The listing builds one solid part. Answer for the finished solid, in the listing's coordinates (mm). A direction names the side the tool comes from. Give positions to 0.01 mm unless a question says otherwise; leave off trailing zeros. Write each loop counter-clockwise with the first axis right and the second up, starting at its lowest first coordinate (ties: lowest second). Pieces come first, ordered by that corner, then holes. Notation, with made-up numbers: (-7, -14) - (16, -14) arc R31 cw to (16, 12) - close; hole circle Ø1 at (0, 5). An arc over 180 degrees is marked (long way). One line per item, written item: value. Start each with the question number.
from build123d import *

# Parameters (mm, degrees)
F1_DEPTH      = 57.15
F1_DEPTH_BACK = 57.15
F2_R          = 6.35
F3_R          = 6.35
F4_R          = 9.525
F5_R          = 4.445
F6_DEPTH      = 101.346
F6_DEPTH_BACK = 150.622
F7_R          = 4.7625
F8_DEPTH      = 25.4
F8_DEPTH_BACK = 25.4
F9_R          = 25.4


with BuildPart() as f1:
    # F0 (on Front) → F1 (new body, two sides)
    with BuildSketch(Plane.XZ) as f1_sk:
        Polygon((-22.225, 0), (0, 0), (22.225, 0), (22.225, 76.2), (19.05, 76.2), (19.05, 3.175), (0, 3.175), (-19.05, 3.175), (-19.05, 76.2), (-22.225, 76.2), align=None)
    extrude(amount=F1_DEPTH)
    extrude(f1_sk.sketch, amount=-F1_DEPTH_BACK)

    # F2
    f2_edges = [f1.edges().sort_by_distance(p)[0] for p in [
        (19.05, 0, 3.175),
    ]]
    fillet(f2_edges, radius=F2_R)

    # F3
    f3_edges = [f1.edges().sort_by_distance(p)[0] for p in [
        (-19.05, 0, 3.175),
    ]]
    fillet(f3_edges, radius=F3_R)

    # F4
    f4_edges = [f1.edges().sort_by_distance(p)[0] for p in [
        (22.225, 0, 0),
        (-22.225, 0, 0),
    ]]
    fillet(f4_edges, radius=F4_R)

    # F5 (on face) → F6 (cut, two sides)
    with BuildSketch(Plane(origin=(-22.225, 0, 0), x_dir=(0, -1, 0), z_dir=(-1, 0, 0))) as f6_sk:
        with Locations((0, 50.8)):
            Circle(F5_R)
    extrude(amount=F6_DEPTH, mode=Mode.SUBTRACT)
    extrude(f6_sk.sketch, amount=-F6_DEPTH_BACK, mode=Mode.SUBTRACT)

    # F7 (on face) → F8 (cut, two sides)
    with BuildSketch(Plane.XY.offset(3.175)) as f8_sk:
        with Locations((0, 31.75)):
            Circle(F7_R)
        with Locations((0, -31.75)):
            Circle(F7_R)
    extrude(amount=F8_DEPTH, mode=Mode.SUBTRACT)
    extrude(f8_sk.sketch, amount=-F8_DEPTH_BACK, mode=Mode.SUBTRACT)

    # F9
    f9_edges = [f1.edges().sort_by_distance(p)[0] for p in [
        (20.6375, 57.15, 76.2),
        (-20.6375, 57.15, 76.2),
        (20.6375, -57.15, 76.2),
        (-20.6375, -57.15, 76.2),
    ]]
    fillet(f9_edges, radius=F9_R)


solid = f1.part
Item 1: Find section B-B on x = 0. Give the number of separate pieces and of enclosed holes in the cut face, plus the area to 3 significant figures.
Item 2: Find section A-A on z = 23.5. Determine the outline of the cut face in (x, y) (3 decimals), plus the area to 3 significant figures.
Item 3: Find section C-C on y = -19. Determine the outline of the cut face in (x, z) (3 decimals), plus the area to 3 significant figures.
Item 4: Straight lines are drawn through the part: line 1 along X through (y, z) = (36, 68) (3 decimals); line 2 along Z through (x, y) = (-20.75, 0) (3 decimals). For each, find the intervals that lie inside material, in ascending order.
Item 5: For faces 1 (the cylindrical face through (-20.66, -49.51, 68.96)), 2 (the cylindrical face through (17.14, -0.8, 4.986)), determine the directions among +Z, -Z, +X, -X, +Y, -Y from which every point of the face is accessible in a straight line to the end or side of a thin tool.
Item 6: Each of these flat-tipped pins is pushed along its axis until it touches: pin 1 Ø1.5 at (x, y) = (5, -25.5) entering from +Z (3 decimals); pin 2 Ø12 at (x, y) = (15, -41.5) entering from +Z. Where does it stop, or does it pass through?
Item 7: Find section D-D on z = 48. Determine the outline of the cut face in (x, y) (3 decimals), plus the area to 3 significant figures.
Item 8: The mould has two halves that part along Y. Classify faces 3 (the cylindrical face through (-20.66, -2.051, 46.857)), 4 (the flat face through (21, 0, 76.2)), 5 (the flat face through (0, -57.15, 3)): +Y half, -Y half, draft (parallel to the pull), parting line (faces both ways), or undercut.
Values:
1. separate pieces: 3
1. enclosed holes: 0
1. area: 302 mm^2
2. outline: (-22.225, -57.15) - (-19.05, -57.15) - (-19.05, 57.15) - (-22.225, 57.15) - close; (19.05, -57.15) - (22.225, -57.15) - (22.225, 57.15) - (19.05, 57.15) - close
2. area: 726 mm^2
3. outline: (-22.225, 9.525) arc R9.525 ccw to (-12.7, 0) - (12.7, 0) arc R9.525 ccw to (22.225, 9.525) - (22.225, 76.2) - (19.05, 76.2) - (19.05, 9.525) arc R6.35 cw to (12.7, 3.175) - (-12.7, 3.175) arc R6.35 cw to (-19.05, 9.525) - (-19.05, 76.2) - (-22.225, 76.2) - close
3. area: 583 mm^2
4. line 1: -22.225 to -19.05, 19.05 to 22.225
4. line 2: 4.434 to 46.355, 55.245 to 76.2
5. face 1: +Z, +X, -X, -Y
5. face 2: +Z, +Y, -Y
6. pin 1: z = 3.175
6. pin 2: z = 75.64
7. outline: (-22.225, -57.15) - (-19.05, -57.15) - (-19.05, -3.452) - (-22.225, -3.452) - close; (-22.225, 3.452) - (-19.05, 3.452) - (-19.05, 57.15) - (-22.225, 57.15) - close; (19.05, -57.15) - (22.225, -57.15) - (22.225, -3.452) - (19.05, -3.452) - close; (19.05, 3.452) - (22.225, 3.452) - (22.225, 57.15) - (19.05, 57.15) - close
7. area: 682 mm^2
8. face 3: undercut
8. face 4: draft
8. face 5: -Y half
